```python
from build123d import *

# Parameters (mm, degrees)
SKETCH1_R           = 2.5
BOSS_EXTRUDE1_DEPTH = 3
CUT_EXTRUDE1_DEPTH  = 1
SKETCH3_R           = 3
CUT_EXTRUDE2_DEPTH  = 38.815340802
CHAMFER1_SIZE       = 0.5
CHAMFER2_SIZE       = 0.5


with BuildPart() as part:
    # Sketch1 → Boss-Extrude1 (new, symmetric)
    with BuildSketch(Plane.XY):
        with BuildLine():
            Line((-31, 6), (31, 6))
            ThreePointArc((31, 6), (37, 0), (31, -6))
            Line((31, -6), (-31, -6))
            ThreePointArc((-31, -6), (-37, 0), (-31, 6))
        make_face()
        with Locations((-31, 0)):
            Circle(SKETCH1_R, mode=Mode.SUBTRACT)
        with Locations((31, 0)):
            Circle(SKETCH1_R, mode=Mode.SUBTRACT)
    extrude(amount=BOSS_EXTRUDE1_DEPTH, both=True)

    # Sketch2 → Cut-Extrude1 (cut)
    with BuildSketch(Plane.XY.offset(3)):
        with BuildLine():
            Line((-26.641101056, 4.75), (26.641101056, 4.75))
            ThreePointArc((26.641101056, 4.75), (27.549994316, 4.167028828), (27.399170438, 3.097826087))
            ThreePointArc((27.399170438, 3.097826087), (26.25, 0), (27.399170438, -3.097826087))
            ThreePointArc((27.399170438, -3.097826087), (27.549994316, -4.167028828), (26.641101056, -4.75))
            Line((26.641101056, -4.75), (-26.641101056, -4.75))
            ThreePointArc((-26.641101056, -4.75), (-27.549994316, -4.167028828), (-27.399170438, -3.097826087))
            ThreePointArc((-27.399170438, -3.097826087), (-26.25, 0), (-27.399170438, 3.097826087))
            ThreePointArc((-27.399170438, 3.097826087), (-27.549994316, 4.167028828), (-26.641101056, 4.75))
        make_face()
    cut_extrude1 = extrude(amount=-CUT_EXTRUDE1_DEPTH, mode=Mode.SUBTRACT)

    # Mirror1: Cut-Extrude1 across plane
    add(cut_extrude1.mirror(Plane.XY), mode=Mode.SUBTRACT)

    # Sketch3 → Cut-Extrude2 (cut, through all)
    with BuildSketch(Plane.XY.offset(2)):
        Circle(SKETCH3_R)
        with Locations((-20, 0)):
            Circle(SKETCH3_R)
        with Locations((-10, 0)):
            Circle(SKETCH3_R)
        with Locations((10, 0)):
            Circle(SKETCH3_R)
        with Locations((20, 0)):
            Circle(SKETCH3_R)
    extrude(amount=-CUT_EXTRUDE2_DEPTH, mode=Mode.SUBTRACT)

    # Chamfer1
    chamfer1_edges = [part.edges().sort_by_distance(p)[0] for p in [
        (-33.5, 0, 3),
        (37, 0, 3),
        (28.5, 0, 3),
        (0, 6, 3),
        (27.549994316, -4.167028828, 3),
        (26.25, 0, 3),
        (27.549994316, 4.167028828, 3),
        (0, 4.75, 3),
        (-27.549994316, 4.167028828, 3),
        (-26.25, 0, 3),
        (-27.549994316, -4.167028828, 3),
        (0, -4.75, 3),
        (-37, 0, 3),
        (17, 0, 2),
        (7, 0, 2),
        (-13, 0, 2),
        (-23, 0, 2),
        (-3, 0, 2),
        (0, -6, 3),
    ]]
    chamfer(chamfer1_edges, length=CHAMFER1_SIZE)

    # Chamfer2
    chamfer2_edges = [part.edges().sort_by_distance(p)[0] for p in [
        (-33.5, 0, -3),
        (28.5, 0, -3),
        (27.549994316, -4.167028828, -3),
        (26.25, 0, -3),
        (0, 6, -3),
        (27.549994316, 4.167028828, -3),
        (0, 4.75, -3),
        (-27.549994316, 4.167028828, -3),
        (-26.25, 0, -3),
        (-27.549994316, -4.167028828, -3),
        (0, -4.75, -3),
        (37, 0, -3),
        (0, -6, -3),
        (-37, 0, -3),
        (17, 0, -2),
        (7, 0, -2),
        (-13, 0, -2),
        (-23, 0, -2),
        (-3, 0, -2),
    ]]
    chamfer(chamfer2_edges, length=CHAMFER2_SIZE)


solid = part.part
```
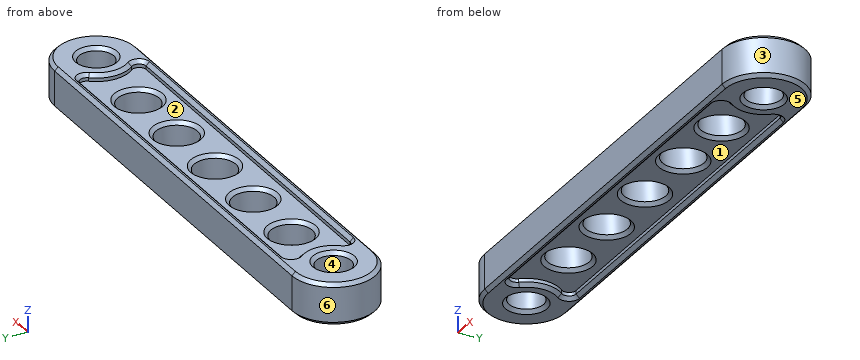
Could you check a few things on this model? Use its own coordinates, in mm. Face numbers are marked on the shaded views. A direction names the side the tool comes from. Round coordinates to 2 decimals unless told otherwise and drop trailing zeros. Loops run counter-clockwise (first coordinate to the right, second up) from the corner with the lowest first, then second, coordinate; pieces in that order, holes last. Notation, with made-up numbers: (28.5, 41) -> (70.5, 41) arc R29 ccw to (70.5, 61) -> close; hole circle Ø7 at (53.25, 70). An arc over 180 degrees is marked (long way). Put each result on its own line as item: value.
Q1. I want a section at B-B on z = 0.75. Write out the boundary of the cut face in (x, y).
Checks:
outline: (-31, -6) -> (31, -6) arc R6 ccw to (31, 6) -> (-31, 6) arc R6 ccw to start; hole circle Ø5 at (-31, 0); hole circle Ø6 at (-20, 0); hole circle Ø6 at (-10, 0); hole circle Ø6 at (0, 0); hole circle Ø6 at (10, 0); hole circle Ø6 at (20, 0); hole circle Ø5 at (31, 0)
Q2. Please list where these lines run through material, in increasing order: line 1 (Y direction, x = -10, z = -0.45); line 2 (Y direction, x = 31, z = 0.75); line 3 (X direction, y = 2.75, z = 0.5). Write a range as from..to.
Checks:
line 1: -6..-3, 3..6
line 2: -6..-2.5, 2.5..6
line 3: -36.33..-21.2, -18.8..-11.2, -8.8..-1.2, 1.2..8.8, 11.2..18.8, 21.2..36.33
Q3. I want a section at C-C on y = 0. Give the number of separate pieces and of enclosed holes in the cut face, and give its area (4 significant figures).
Checks:
separate pieces: 8
enclosed holes: 0
area: 154.5 mm2
Q4. For pin 1 Ø1.5 at (y, z) = (-4.5, 0) entering from -X; pin 2 Ø1 at (y, z) = (1, -1.5) entering from +X; pin 3 Ø3 at (x, y) = (31, 0) entering from -Z; pin 4 Ø5 at (x, y) = (-0.5, 0.5) entering from +Z, each with a flat end and sliding along its axis, tell me the tip position at first contact or that it passes through.
Checks:
pin 1: x = -35.68
pin 2: x = 36.98
pin 3: through
pin 4: z = 1.71
Q5. I want a section at A-A on x = 20. Write out the boundary of the cut face in (y, z), and give its area (3 significant figures).
Checks:
outline: (-6, -2.5) -> (-5.5, -3) -> (-5.25, -3) -> (-4.75, -2.5) -> (-4.75, -2) -> (-3.5, -2) -> (-3, -1.5) -> (-3, 1.5) -> (-3.5, 2) -> (-4.75, 2) -> (-4.75, 2.5) -> (-5.25, 3) -> (-5.5, 3) -> (-6, 2.5) -> close; (3, -1.5) -> (3.5, -2) -> (4.75, -2) -> (4.75, -2.5) -> (5.25, -3) -> (5.5, -3) -> (6, -2.5) -> (6, 2.5) -> (5.5, 3) -> (5.25, 3) -> (4.75, 2.5) -> (4.75, 2) -> (3.5, 2) -> (3, 1.5) -> close
area: 27.5 mm2
Q6. Which directions (+Z, -Z, +X, -X, +Y, -Y) give clear straight access to the entire face, cutting with the end or side of a thin tool? Please do the marked faces 1, 2 and 3.
Checks:
face 1: -Z
face 2: +Z
face 3: +Z, -Z, +X
Q7. Thinking about a two-plate mould opening in X: for the marked faces 4, 5 and 6, which applies, pulls with the +X half, pulls with the -X half, needs draft (parallel to the pull), parting line crosses it, or undercut?
Checks:
face 4: undercut
face 5: needs draft
face 6: pulls with the -X half
Q8. I want a section at D-D on x = -24.5. Write out the boundary of the cut face in (y, z).
Checks:
outline: (-6, -2.5) -> (-5.5, -3) -> (-5.25, -3) -> (-4.75, -2.5) -> (-4.75, -2) -> (4.75, -2) -> (4.75, -2.5) -> (5.25, -3) -> (5.5, -3) -> (6, -2.5) -> (6, 2.5) -> (5.5, 3) -> (5.25, 3) -> (4.75, 2.5) -> (4.75, 2) -> (-4.75, 2) -> (-4.75, 2.5) -> (-5.25, 3) -> (-5.5, 3) -> (-6, 2.5) -> close
